Here's how the part is built. I have some questions about the finished solid (model axes, mm). A direction names the side the tool comes from. Give positions to 0.01 mm unless a question says otherwise; leave off trailing zeros. Loops run counter-clockwise (first coordinate to the right, second up) from the corner with the lowest first, then second, coordinate; pieces in that order, holes last. Notation, with made-up numbers: (-39, -15) - (10, -15) arc R28 cw to (10, 6) - close; hole circle Ø9 at (69.25, 50.25). An arc over 180 degrees is marked (long way). Use one line per item in the form item = value.
from build123d import *

# Parameters (mm, degrees)
SKETCH_5_R           = 31
EXTRUDE_4_DEPTH      = 10
SKETCH_6_R           = 3
CUT_EXTRUDE_5_DEPTH  = 10
SKETCH_8_R           = 17.5
EXTRUDE_5_DEPTH      = 90
SKETCH_4_R           = 12.5
CUT_EXTRUDE_6_DEPTH  = 88
CUT_EXTRUDE_10_DEPTH = 120


with BuildPart() as part:
    # Sketch 5 → Extrude 4 (new body)
    with BuildSketch(Plane.XY):
        Circle(SKETCH_5_R)
    extrude(amount=EXTRUDE_4_DEPTH)

    # Sketch 6 → Cut-Extrude 5 (cut)
    with BuildSketch(Plane.XY):
        with Locations((0, -25)):
            Circle(SKETCH_6_R)
        with Locations((-25, 0)):
            Circle(SKETCH_6_R)
        with Locations((0, 25)):
            Circle(SKETCH_6_R)
        with Locations((25, 0)):
            Circle(SKETCH_6_R)
    extrude(amount=CUT_EXTRUDE_5_DEPTH, mode=Mode.SUBTRACT)

    # Sketch 8 → Extrude 5 (add)
    with BuildSketch(Plane.XY):
        with Locations(Location((0, 0, 0), (0, 0, 180))):
            Circle(SKETCH_8_R)
    extrude(amount=EXTRUDE_5_DEPTH)

    # Sketch 4 → Cut-Extrude 6 (cut)
    with BuildSketch(Plane.XY):
        Circle(SKETCH_4_R)
    extrude(amount=CUT_EXTRUDE_6_DEPTH, mode=Mode.SUBTRACT)

    # Sketch 12 → Cut-Extrude 10 (cut)
    with BuildSketch(Plane.XY):
        Polygon((8.640186366, -16.018650991), (-15.798690834, 9.036114648), (-8.640186366, 16.018650991), (15.798690834, -9.036114648), align=None)
    extrude(amount=CUT_EXTRUDE_10_DEPTH, mode=Mode.SUBTRACT)


solid = part.part
(1) Thinking about a two-plate mould opening in X: for faces 4 (the flat face through (13, -13, 10)), 5 (the cylindrical face through (-28, 0, 5)), 6 (the cylindrical face through (12.745, 11.993, 49.44)), which applies, pulls with the +X half, pulls with the -X half, needs draft (parallel to the pull), parting line crosses it, or undercut?
Geometry says:
face_4 = needs draft
face_5 = undercut
face_6 = parting line crosses it
(2) For P1, Ø10, axis at x = 4.5, z = 55, coming from the -Y side; P2, Ø2, axis at y = 3.5, z = 44, coming from the +X side; P3, Ø6, axis at y = -4, z = 80.5, coming from the +X side; P4, Ø5.5, axis at x = 0, y = -25, coming from the +Z side, each with a flat end and sliding along its axis, tell me the tip position at first contact or that it passes through.
Geometry says:
P1 = -17.5
P2 = 17.32
P3 = 17.47
P4 = through
(3) If we section it at D-D (x = 0): List the corners of the cut face in (y, z) for me, plus the area to 3 significant figures.
Geometry says:
outline = (-31, 0) - (-28, 0) - (-28, 10) - (-31, 10) - close; (-22, 0) - (-12.5, 0) - (-12.5, 88) - (-7.16, 88) - (-7.16, 90) - (-17.5, 90) - (-17.5, 10) - (-22, 10) - close; (7.16, 88) - (12.5, 88) - (12.5, 0) - (22, 0) - (22, 10) - (17.5, 10) - (17.5, 90) - (7.16, 90) - close; (28, 0) - (31, 0) - (31, 10) - (28, 10) - close
area = 1,070 mm²
(4) For faces 1 (the flat face through (-12.27, 12.48, 4.93)), 2 (the cylindrical face through (-9.09, -8.58, 43.38)), 3 (the cylindrical face through (-12.745, -11.993, 49.44)), which set-ups out of +Z, -Z, +X, -X, +Y, -Y let a thin tool reach every point of the face, with its end or its side?
Geometry says:
face_1 = +Z, -Z
face_2 = -Z
face_3 = +Z
(5) If we section it at A-A (x = 14): List the corners of the cut face in (y, z) for me.
Geometry says:
outline = (-27.66, 0) - (-10.79, 0) - (-10.79, 10) - (-27.66, 10) - close; (-7.19, 0) - (27.66, 0) - (27.66, 10) - (10.5, 10) - (10.5, 90) - (-7.19, 90) - close
(6) If I drill on probe 1 along Y at (x, z) = (0, 4.75); probe 2 along X at (y, z) = (4, 8); probe 3 along Z at (x, y) = (-10, 22.5), over which ranges is the centre line in solid material (lowest first)?
Geometry says:
probe_1 = -31 to -28, -22 to -12.5, 12.5 to 22, 28 to 31
probe_2 = -30.74 to -11.84, 11.84 to 30.74
probe_3 = 0 to 10
(7) If we section it at B-B (y = 25): List the corners of the cut face in (x, z) for me, plus the area to 3 significant figures.
Geometry says:
outline = (-18.33, 0) - (-3, 0) - (-3, 10) - (-18.33, 10) - close; (3, 0) - (18.33, 0) - (18.33, 10) - (3, 10) - close
area = 307 mm²
(8) If we section it at C-C (y = 0): List the corners of the cut face in (x, z) for me, plus the area to 3 significant figures.
Geometry says:
outline = (-31, 0) - (-28, 0) - (-28, 10) - (-31, 10) - close; (-22, 0) - (-12.5, 0) - (-12.5, 88) - (-6.98, 88) - (-6.98, 90) - (-17.5, 90) - (-17.5, 10) - (-22, 10) - close; (6.98, 88) - (12.5, 88) - (12.5, 0) - (22, 0) - (22, 10) - (17.5, 10) - (17.5, 90) - (6.98, 90) - close; (28, 0) - (31, 0) - (31, 10) - (28, 10) - close
area = 1,070 mm²
